from build123d import *
from build123d import SkipClean  # not in build123d's __all__

# Parameters (mm, degrees)
F1_DEPTH    = 10
F3_R        = 5
F4_R        = 3
F5_R        = 2
F7_DEPTH    = 10.0010001
F8_T1_DEPTH = 10


# Not quite as in the source:
# - a fillet or chamfer that OpenCascade refuses, or shapes differently, is made with other operations: its cross-section is extruded or revolved along the edge and cut away or added


with BuildPart() as f1:
    # F0 (on Front) → F1 (new body)
    with BuildSketch(Plane.XZ):
        with BuildLine():
            ThreePointArc((-60, 9), (-57.6213157363, 8.9328971517), (-55.2831757887, 8.4904683961))
            ThreePointArc((-55.2831757887, 8.4904683961), (-45.1436514688, 8.7416176388), (-40, 0))
            ThreePointArc((-40, 0), (-41.6794970566, -5.5470019623), (-46.1538461538, -9.2307692308))
            ThreePointArc((-46.1538461538, -9.2307692308), (-25.4921003461, -2.7389543798), (-4, -0.0666851955))
            ThreePointArc((-4, -0.0666851955), (-4.6347028183, 2.6231856146), (-5.9814434357, 5.03659448))
            ThreePointArc((-5.9814434357, 5.03659448), (-6.715086481, 12.9015322824), (0, 17.061230866))
            Line((0, 17.061230866), (0, 22.061230866))
            ThreePointArc((0, 22.061230866), (-30.1526886016, 20.5420767676), (-60, 16))
            Line((-60, 16), (-60, 9))
        make_face()
        with BuildLine():
            ThreePointArc((-46.6427971379, 2.1746698468), (-46.1640639051, 1.1338404984), (-46, 0))
            ThreePointArc((-46, 0), (-48.9877288652, -3.8697941999), (-53.4876535749, -1.958640483))
            ThreePointArc((-53.4876535749, -1.958640483), (-55.921777017, 1.4722128283), (-59.0196729824, 4.3180434563))
            ThreePointArc((-59.0196729824, 4.3180434563), (-59.7518390528, 2.21396366), (-60, 0))
            ThreePointArc((-60, 0), (-55.5470019623, -8.3205029434), (-46.1538461538, -9.2307692308))
            ThreePointArc((-46.1538461538, -9.2307692308), (-41.6794970566, -5.5470019623), (-40, 0))
            ThreePointArc((-40, 0), (-45.1436514688, 8.7416176388), (-55.2831757887, 8.4904683961))
            ThreePointArc((-55.2831757887, 8.4904683961), (-50.3805281419, 6.1294058803), (-46.6427971379, 2.1746698468))
        make_face()
        with BuildLine():
            ThreePointArc((-5.9814434357, 5.03659448), (-4.6347028183, 2.6231856146), (-4, -0.0666851955))
            ThreePointArc((-4, -0.0666851955), (-2.0002779129, -0.0166724571), (0, 0))
            Line((0, 0), (0, 2.061230866))
            ThreePointArc((0, 2.061230866), (-3.3403014164, 2.846144385), (-5.9814434357, 5.03659448))
        make_face()
    extrude(amount=F1_DEPTH)

    # F2: F1 across plane


with BuildPart() as f1_1:
    add(f1.part, clean=False)
    with SkipClean():  # cleaning this boolean's faces spoils the solid; the shape is the same uncleaned
        add(f1.part.mirror(Plane.YZ), clean=False)

    # F3
    f3_edges = [f1_1.edges().sort_by_distance(p)[0] for p in [
        (-60, -5, 16),
        (60, -5, 16),
    ]]
    fillet(f3_edges, radius=F3_R)

    # F4
    f4_edges = [f1_1.edges().sort_by_distance(p)[0] for p in [
        (-60, -5, 9),
        (60, -5, 9),
    ]]
    fillet(f4_edges, radius=F4_R)

    # F5
    f5_edges = [f1_1.edges().sort_by_distance(p)[0] for p in [
        (-59.019673, -5, 4.318043),
        (59.019673, -5, 4.318043),
    ]]
    fillet(f5_edges, radius=F5_R)

    # F6 (on face) → F7 (cut, through all)
    with BuildSketch(Plane.XZ.offset(10)):
        with BuildLine():
            ThreePointArc((-7.8234196702, 2.7509433962), (-12.1811976175, 9.6949287705), (-11.2993718648, 17.8454836508))
            ThreePointArc((-11.2993718648, 17.8454836508), (-33.2415394106, 16.1887543276), (-55, 12.9065505808))
            ThreePointArc((-55, 12.9065505808), (-44.9636385736, 6.903343626), (-40, -3.685770432))
            ThreePointArc((-40, -3.685770432), (-24.1273224471, 0.6104154355), (-7.8234196702, 2.7509433962))
        make_face()
        with BuildLine():
            ThreePointArc((40, -3.685770432), (42.6359894717, 6.412330531), (50, 13.8076961402))
            ThreePointArc((50, 13.8076961402), (30.7161061945, 16.4632023612), (11.2993718648, 17.8454836508))
            ThreePointArc((11.2993718648, 17.8454836508), (12.1961499726, 15.2393294517), (12.5, 12.5))
            ThreePointArc((12.5, 12.5), (11.2703759005, 7.0936493768), (7.8234196702, 2.7509433962))
            ThreePointArc((7.8234196702, 2.7509433962), (24.1273224471, 0.6104154355), (40, -3.685770432))
        make_face()
    extrude(amount=-F7_DEPTH, mode=Mode.SUBTRACT)

    # F8: fillet of radius 8 on 8 edges, made by hand

    # F8_s2 → F8_t1 (join)
    with BuildSketch(Plane.XZ):
        with BuildLine():
            ThreePointArc((-36.7451179027, 15.7716261712), (-42.9406323526, 11.3440144515), (-42.6227863201, 3.7356559729))
            ThreePointArc((-42.6227863201, 3.7356559729), (-47.8930149535, 9.5605639606), (-55, 12.9065505808))
            ThreePointArc((-55, 12.9065505808), (-45.8949216066, 14.4815724477), (-36.7451179027, 15.7716261712))
        make_face()
        with BuildLine():
            ThreePointArc((-42.0039790926, 2.6185161763), (-38.1014001727, -1.0557269801), (-32.7552534978, -1.4416035521))
            ThreePointArc((-32.7552534978, -1.4416035521), (-36.3949282061, -2.5078334489), (-40, -3.685770432))
            ThreePointArc((-40, -3.685770432), (-40.7395345489, -0.4501990795), (-42.0039790926, 2.6185161763))
        make_face()
        with BuildLine():
            ThreePointArc((-12.3583566886, 10.623561896), (-13.8147498473, 4.6940719377), (-19.0299825284, 1.5189687455))
            ThreePointArc((-19.0299825284, 1.5189687455), (-13.4408237395, 2.2634215831), (-7.8234196702, 2.7509433962))
            ThreePointArc((-7.8234196702, 2.7509433962), (-10.83146134, 6.2606534605), (-12.3583566886, 10.623561896))
        make_face()
        with BuildLine():
            ThreePointArc((-12.3513599638, 10.578046035), (-15.2694424, 15.6035487131), (-20.8189034057, 17.3281834039))
            ThreePointArc((-20.8189034057, 17.3281834039), (-16.0612204229, 17.6251616805), (-11.2993718648, 17.8454836508))
            ThreePointArc((-11.2993718648, 17.8454836508), (-12.3710626618, 14.2907564373), (-12.3513599638, 10.578046035))
        make_face()
        with BuildLine():
            ThreePointArc((20.8189034057, 17.3281834039), (15.2694424, 15.6035487131), (12.3513599638, 10.578046035))
            ThreePointArc((12.3513599638, 10.578046035), (12.3710626618, 14.2907564373), (11.2993718648, 17.8454836508))
            ThreePointArc((11.2993718648, 17.8454836508), (16.0612204229, 17.6251616805), (20.8189034057, 17.3281834039))
        make_face()
        with BuildLine():
            ThreePointArc((12.3583566886, 10.623561896), (13.8147498473, 4.6940719377), (19.0299825284, 1.5189687455))
            ThreePointArc((19.0299825284, 1.5189687455), (13.4408237395, 2.2634215831), (7.8234196702, 2.7509433962))
            ThreePointArc((7.8234196702, 2.7509433962), (10.83146134, 6.2606534605), (12.3583566886, 10.623561896))
        make_face()
        with BuildLine():
            ThreePointArc((41.7652662923, 4.7039127832), (41.4390880083, 11.9220711187), (35.429216879, 15.9332618444))
            ThreePointArc((35.429216879, 15.9332618444), (42.7278279524, 14.9610989412), (50, 13.8076961402))
            ThreePointArc((50, 13.8076961402), (45.1669008636, 9.9032127448), (41.7652662923, 4.7039127832))
        make_face()
        with BuildLine():
            ThreePointArc((41.3345230553, 3.6720037672), (37.4981716447, -0.5831636355), (31.800316666, -1.1819043245))
            ThreePointArc((31.800316666, -1.1819043245), (35.9219808015, -2.3623729613), (40, -3.685770432))
            ThreePointArc((40, -3.685770432), (40.3203276581, 0.056042117), (41.3345230553, 3.6720037672))
        make_face()
    extrude(amount=F8_T1_DEPTH)


solid = f1_1.part
Geometry check sheet. Reference: the model listing, model coordinates, mm. A direction names the side the tool comes from. Give positions to 0.01 mm unless a question says otherwise; leave off trailing zeros. Loops run counter-clockwise (first coordinate to the right, second up) from the corner with the lowest first, then second, coordinate; pieces in that order, holes last. Notation, with made-up numbers: M 88,-35.75 L 98,-35.75 A8 ccw 98,-30.75 Z; hole C 84,15.25 d4. An arc over 180 degrees is marked long. Write each question's results on one line, items separated by ' | '.
1) Release check for a two-part mould opening along X. For faces 4 (the face through (59.27, -5.07, 9.92)), 5 (the face through (1, -10, 21)), 6 (the face through (-13.77, -4.93, 4.756)) record: +X half, -X half, draft (parallel to the pull), parting line (faces both ways), or undercut.
Answers follow:
face 4: +X half | face 5: draft | face 6: undercut
2) Tool access check on faces 1 (the face through (41.49, -4.93, 11.83)), 2 (the face through (-59.27, -5.07, 9.92)), 3 (the face through (1, 0, 21)). Record the directions out of +Z, -Z, +X, -X, +Y, -Y that give a thin tool (end or side, any length) a straight path to the whole face; none if there is none.
Answers follow:
face 1: +Y, -Y | face 2: -X, +Y, -Y | face 3: +Z, -Z, +X, -X, +Y
3) Section check C-C, the plane y = -7.75. Count the separate pieces of the cut face and the enclosed holes in it, plus the area to 3 significant figures.
Answers follow:
separate pieces: 1 | enclosed holes: 3 | area: 1,590 mm2
4) Gauge pin test, flat ends, axial feed: pin 1 (2 mm diameter, centred on y = -2, z = 9, fed in from -X); pin 2 (6 mm diameter, centred on x = -4, y = -7.5, fed in from +Z); pin 3 (1.5 mm diameter, centred on y = -5, z = -1, fed in from +X). Record the tip position at first contact, or that the pin passes through.
Answers follow:
pin 1: x = -59.34 | pin 2: z = 22.06 | pin 3: x = 60
5) Section check A-A, the plane x = 23.5. Record the boundary of the cut face in (y, z), plus the area to 3 significant figures.
Answers follow:
outline: M -10,-2.32 L 0,-2.32 L 0,0.73 L -10,0.73 Z; M -10,17.13 L 0,17.13 L 0,21.14 L -10,21.14 Z | area: 70.7 mm2
6) Thickness scan on line 1 (X direction, y = -7, z = 11); line 2 (X direction, y = -9.5, z = 12); line 3 (Z direction, x = 37.5, y = -2). Record the ranges inside material, lowest first.
Answers follow:
line 1: -59.87 to -43.1, -12.43 to -7.36, 7.36 to 12.43, 41.88 to 59.87 | line 2: -60 to -42.58, -12.71 to -7.09, 7.09 to 12.71, 41.39 to 60 | line 3: -6.01 to -0.58, 15.4 to 19.71
7) Section check B-B, the plane z = 7. Record the boundary of the cut face in (x, y), plus the area to 3 significant figures.
Answers follow:
outline: M -51.71,-10 L -43.71,-10 L -43.71,0 L -51.71,0 Z; M -12.64,-10 L -7.05,-10 L -7.05,0 L -12.64,0 Z; M 7.05,-10 L 12.64,-10 L 12.64,0 L 7.05,0 Z; M 42.41,-10 L 51.71,-10 L 51.71,0 L 42.41,0 Z | area: 285 mm2
8) Section check D-D, the plane z = 13. Record the boundary of the cut face in (x, y), plus the area to 3 significant figures.
Answers follow:
outline: M -59.87,-10 L -41.86,-10 L -41.86,0 L -59.87,0 Z; M -13.14,-10 L -6.67,-10 L -6.67,0 L -13.14,0 Z; M 6.67,-10 L 13.14,-10 L 13.14,0 L 6.67,0 Z; M 40.71,-10 L 59.87,-10 L 59.87,0 L 40.71,0 Z | area: 501 mm2
